from build123d import *

# Parameters (mm, degrees)
BOSS_EXTRUDE1_DEPTH = 16.51
SKETCH4_W           = 4.826
SKETCH4_H           = 8.89
BOSS_EXTRUDE2_DEPTH = 6.604
CUT_EXTRUDE1_DEPTH  = 7.874
CIRPATTERN1_COUNT   = 3
BOSS_EXTRUDE3_START = -23.29
BOSS_EXTRUDE3_DEPTH = 3


with BuildPart() as part:
    # Sketch1 → Revolve1 (revolve)
    with BuildSketch(Plane(origin=(0, 0, 0), x_dir=(0, 0, -1), z_dir=(1, 0, 0))):
        Polygon((0, 0), (0, 17.399), (24.5872, 17.399), (24.5872, 14.9225), (83.9978, 14.9225), (83.9978, 0), align=None)
    revolve(axis=Axis((0, 0, 55), (0, 0, -1)))

    # Sketch3 → Boss-Extrude1 (add)
    with BuildSketch(Plane(origin=(0, 0, -83.9978), x_dir=(-1, 0, 0), z_dir=(0, 0, -1))):
        with BuildLine():
            Line((-16.51, 0), (-16.51, 26.035))
            Line((-16.51, 26.035), (16.51, 26.035))
            Line((16.51, 26.035), (16.51, 0))
            ThreePointArc((16.51, 0), (0, -16.51), (-16.51, 0))
        make_face()
    extrude(amount=BOSS_EXTRUDE1_DEPTH)

    # Sketch4 → Boss-Extrude2 (add, symmetric)
    with BuildSketch(Plane(origin=(0, 0, 0), x_dir=(0, 0, -1), z_dir=(1, 0, 0))):
        with Locations((92.7608, 30.48)):
            Rectangle(SKETCH4_W, SKETCH4_H)
    extrude(amount=BOSS_EXTRUDE2_DEPTH, both=True)

    # Sketch5 → Revolve2 (revolve)
    with BuildSketch(Plane(origin=(0, 0, 0), x_dir=(0, 0, -1), z_dir=(1, 0, 0))):
        Polygon((0, 13.0048), (-1.524, 13.0048), (-1.524, 9.0297), (-19.05, 9.0297), (-19.05, 6.6548), (0, 6.6548), align=None)
    revolve(axis=Axis((0, 6.6548, 5.02539), (0, 0, -1)))

    # Sketch6 → Cut-Extrude1 (cut)
    with BuildSketch(Plane.XY.offset(19.05)):
        with BuildLine():
            Line((-1.669458355, 8.3439), (1.669458355, 8.3439))
            ThreePointArc((1.669458355, 8.3439), (0, 9.0297), (-1.669458355, 8.3439))
        make_face()
    extrude(amount=-CUT_EXTRUDE1_DEPTH, mode=Mode.SUBTRACT)

    # Sketch7 → #4-40 Tapped Hole1 (revolve, cut)
    with BuildSketch(Plane(origin=(3.49243949, -13.033961618, 0), x_dir=(0, -1, 0), z_dir=(1, 0, 0))):
        Polygon((0, 0), (0, 7.409152758), (1.1303, 6.73), (1.1303, 0), align=None)
    f_4_40_tapped_hole1 = revolve(axis=Axis((3.49243949, -13.033961618, 6.35), (0, 0, -1)), mode=Mode.SUBTRACT)

    # CirPattern1: #4-40 Tapped Hole1 ×3 about axis
    cirpattern1_axis = Axis((0, 0, 0), (0, 0, 1))
    for i in range(1, CIRPATTERN1_COUNT):
        add(f_4_40_tapped_hole1.rotate(cirpattern1_axis, i * 360 / CIRPATTERN1_COUNT), mode=Mode.SUBTRACT)

    # Sketch9 → Boss-Extrude3 (add)
    with BuildSketch(Plane(origin=(0, 0, -100.5078), x_dir=(-1, 0, 0), z_dir=(0, 0, -1)).offset(BOSS_EXTRUDE3_START)):
        Polygon((0, 0), (-1.922523392, 0.551274712), (7.724784062, 34.195434069), (11.569830845, 33.092884646), (1.922523392, -0.551274712), align=None)
    extrude(amount=-BOSS_EXTRUDE3_DEPTH)


solid = part.part
The listing builds one solid part. Answer for the finished solid, in the listing's coordinates (mm). A direction names the side the tool comes from. Round coordinates to 2 decimals unless told otherwise and drop trailing zeros. Order: outer loops, then holes, each group sorted by start corner. A loop starts at its lowest first (then second) coordinate and runs counter-clockwise, first axis right, second up. Notation, with made-up numbers: M -9,-30 L 2,-30 A11 cw 2,-14 Z; hole C -14.75,-38 d9. An arc over 180 degrees is marked long. Answer in a Markdown table with one row per item. Add a question column.
1) The part is cut by section C-C on z = -44. Determine the outline of the cut face in (x, y) (1 decimal).
2) Determine the mould class of faces 5 (the face through (-0.363, -16.506, -92.137)), 6 (the face through (0.1, 9.4, 1.524)), 7 (the face through (-9.62, 33.65, -75.74)), 8 (the face through (2.73, -12.2, -3.32)) for opening direction Y: pulls with the +Y half, pulls with the -Y half, needs draft (parallel to the pull), parting line crosses it, or undercut.
3) Flat-ended cylindrical pins translate along their axes: pin 1 Ø4 at (y, z) = (30.5, -93.5) entering from -X; pin 2 Ø4 at (y, z) = (-12, -44) entering from -X; pin 3 Ø4 at (x, z) = (-6.5, -48) entering from +Y. Find the tip coordinate at first contact, or state that the pin passes through.
4) The part is cut by section D-D on y = -6. Determine the outline of the cut face in (x, z), plus the area to 3 significant figures.
5) The part is cut by section A-A on y = 29.5. Determine the outline of the cut face in (x, z), plus the area to 3 significant figures.
6) Which of the six approach directions +Z, -Z, +X, -X, +Y, -Y give full straight-line access (tool end or side, diameter ignored) to faces 1 (the face through (16.51, 13, -92)), 2 (the face through (-13.987, 2.885, -3.318)), 3 (the face through (-4, 15, -83.998)), 4 (the face through (6.604, 31, -93))?
7) Consider line 1 along Z through (x, y) = (-9.5, 7); line 2 along X through (y, z) = (10.5, -91.5); line 3 along Z through (x, y) = (0, 8.5). Determine where each line is inside the solid, lowest interval first. Write a range as from..to.
Findings below:
| question | item | result |
|---|---|---|
| 1 | outline | C 0,0 d29.8 |
| 2 | face 5 | pulls with the -Y half |
| 2 | face 6 | needs draft |
| 2 | face 7 | pulls with the +Y half |
| 2 | face 8 | undercut |
| 3 | pin 1 | stops at x = -6.6 |
| 3 | pin 2 | stops at x = -11.08 |
| 3 | pin 3 | stops at y = 14.23 |
| 4 | outline | M -16.33,-24.59 L -13.66,-24.59 L -13.66,-84 L -15.38,-84 L -15.38,-100.51 L 15.38,-100.51 L 15.38,-84 L 13.66,-84 L 13.66,-24.59 L 16.33,-24.59 L 16.33,0 L -16.33,0 Z |
| 4 | area | 2,930 mm² |
| 5 | outline | M -10.54,-77.22 L -6.38,-77.22 L -6.38,-74.22 L -10.54,-74.22 Z; M -6.6,-95.17 L 6.6,-95.17 L 6.6,-90.35 L -6.6,-90.35 Z |
| 5 | area | 76.2 mm² |
| 6 | face 1 | -Z, +X, +Y, -Y |
| 6 | face 2 | +Z |
| 6 | face 3 | none |
| 6 | face 4 | +Z, -Z, +X, +Y |
| 7 | line 1 | z = -100.51..0 |
| 7 | line 2 | x = -16.51..16.51 |
| 7 | line 3 | z = -100.51..11.18 |
